Autodesk Fusion 360 part; units mm, degrees
sketch "草图1" plane through (0, 0, 0) normal (0, 0, 1) x (1, 0, 0)
  line L0 (-100, 87.5) -> (100, 87.5)
  line L1 (100, 87.5) -> (100, -87.5)
  line L2 (100, -87.5) -> (-100, -87.5)
  line L3 (-100, -87.5) -> (-100, 87.5)
  line L4 (-100, 0) -> (100, 0) construction
  line L5 (0, 75) -> (0, -50) construction
  dimension "d1" = 200
  dimension "d2" = 175
extrude "拉伸1" add sketch "草图1" against normal blind 100
sketch "草图2" plane through (0, -87.5, 0) normal (0, -1, 0) x (1, 0, 0)
  line L0 (100, 0) -> (-100, 0)
  line L1 (-100, 0) -> (-100, -100)
  line L2 (-100, -100) -> (100, -100)
  line L3 (100, -100) -> (100, 0)
  circle A0 centre (0, 0) radius 50
  dimension "d5" = 100
extrude "拉伸2" cut sketch "草图2" against normal blind 100 contours L0 A0 picked at (10.3915, -13.0305)
sketch "草图3" plane through (100, 0, 0) normal (1, 0, 0) x (0, 1, 0)
  line L0 (87.5, 0) -> (-87.5, 0)
  line L1 (-87.5, 0) -> (-87.5, -100)
  line L2 (-87.5, -100) -> (87.5, -100)
  line L3 (87.5, -100) -> (87.5, 0)
  line L4 (87.5, 0) -> (312.5, -75)
  line L5 (312.5, -75) -> (312.5, -100)
  line L6 (312.5, -100) -> (87.5, -100)
  line L7 (-150, 0) -> (245.1978, 0) construction
  dimension "d8" = 25
  dimension "d9" = 225
extrude "拉伸3" add sketch "草图3" against normal blind 100 contours L3 L4 L5 L6
sketch "草图4" plane through (-100, 0, 0) normal (-1, 0, 0) x (0, -1, 0)
  line L0 (87.5, 0) -> (-87.5, 0)
  line L1 (-87.5, 0) -> (-87.5, -100)
  line L2 (-87.5, -100) -> (87.5, -100)
  line L3 (87.5, -100) -> (87.5, 0)
  line L4 (-312.5, 75) -> (-87.5, 0)
  line L5 (-87.5, -100) -> (-312.5, -100)
  line L6 (-312.5, -100) -> (-312.5, 75)
  dimension "d12" = 175
  dimension "d13" = 225
extrude "拉伸4" add sketch "草图4" against normal blind 100 contours L1 L4 L5 L6
ref_plane "工作平面1" through (0, 0, 100) normal (0, 0, 1) x (1, 0, 0)
sketch "草图5" plane through (0, 0, 100) normal (0, 0, 1) x (1, 0, 0)
  line L0 (-50, 312.5) -> (50, 312.5)
  line L1 (50, 312.5) -> (0, 37.5)
  line L2 (0, 37.5) -> (-50, 312.5)
  line L3 (0, -125) -> (0, 391.0284) construction
  point P0 (100, -87.5)
  point P1 (-100, -87.5)
  point P2 (-100, 87.5)
  point P3 (100, 87.5)
  point P4 (-100, 312.5)
  point P5 (100, 312.5)
  dimension "d17" = 275
  dimension "d18" = 100
extrude "拉伸5" add sketch "草图5" against normal through all
sketch "草图6" plane through (100, 0, 0) normal (1, 0, 0) x (0, 1, 0)
  line L0 (87.5, 0) -> (-87.5, 0)
  line L1 (-87.5, 0) -> (-87.5, -100)
  line L2 (-87.5, -100) -> (312.5, -100)
  line L3 (312.5, -100) -> (312.5, -75)
  line L4 (312.5, -75) -> (87.5, 0)
  line L5 (37.5, 100) -> (37.5, 93.4578)
  line L6 (37.5, 93.4578) -> (37.5, 75)
  line L7 (37.5, 75) -> (312.5, 100)
  line L8 (312.5, 100) -> (37.5, 100)
  point P0 (37.5, 100)
  point P1 (312.5, 100)
  dimension "d20" = 25
extrude "拉伸6" cut sketch "草图6" against normal blind 375 contours L5 L6 L7 L8
equation "d2 = 400 mm - 225 mm"
Read the model definition and answer for the solid it produces. Units are mm, in the model's axes. A direction names the side the tool comes from. Give positions to 0.01 mm unless a question says otherwise; leave off trailing zeros. Write each loop counter-clockwise with the first axis right and the second up, starting at its lowest first coordinate (ties: lowest second). Pieces come first, ordered by that corner, then holes. Notation, with made-up numbers: (1, 38) - (48, 38) arc R18 cw to (48, 69) - close; hole circle Ø7 at (-21.5, 27). An arc over 180 degrees is marked (long way). Return JSON: item names as keys, results as strings.
Q1. A cutting plane is placed at C-C, the plane z = -46. Determine the outline of the cut face in (x, y).
Reply:
{"outline": "(-100, -87.5) - (-19.6, -87.5) - (-19.6, 12.5) - (19.6, 12.5) - (19.6, -87.5) - (100, -87.5) - (100, 225.5) - (34.18, 225.5) - (50, 312.5) - (-100, 312.5) - close"}
Q2. A cutting plane is placed at B-B, the plane x = 28.5. Determine the outline of the cut face in (y, z).
Reply:
{"outline": "(-87.5, -100) - (194.25, -100) - (194.25, -101) - (312.5, -101) - (312.5, 100) - (194.25, 89.25) - (194.25, -35.58) - (87.5, 0) - (12.5, 0) - (12.5, -41.08) - (-87.5, -41.08) - close"}
Q3. For a pull along Y with two mould halves and no side action, classify faces 1 (the face through (-1, 21, 0)), 2 (the face through (25.35, 176.92, -100.49)), 3 (the face through (65.283, 198.425, -36.975)), 4 (the face through (30.906, 207.481, 33.169)) as released by +Y, released by -Y, zero draft, split by the parting line, or undercut.
Reply:
{"face 1": "zero draft", "face 2": "released by -Y", "face 3": "undercut", "face 4": "undercut"}
Q4. For faces 5 (the face through (-1.099, -38.2, -49.988)), 6 (the face through (-24, 110, -100)), 7 (the face through (-24.65, 173.08, -100.49)), 8 (the face through (-65.283, 201.575, 38.025)), determine the directions among +Z, -Z, +X, -X, +Y, -Y from which every point of the face is accessible in a straight line to the end or side of a thin tool.
Reply:
{"face 5": "+Z, -Y", "face 6": "-Z, -Y", "face 7": "-Z, -X, -Y", "face 8": "+Z, -X, -Y"}
Q5. Consider line 1 along Z through (x, y) = (11, 33); line 2 along Y through (x, z) = (19.5, -46); line 3 along Z through (x, y) = (-3, -48). Determine where each line is inside the solid, lowest interval first. Write a range as [from, to].
Reply:
{"line 1": "[-100, 0]", "line 2": "[12.5, 312.5]", "line 3": "[-100, -49.91]"}
Q6. A cutting plane is placed at D-D, the plane z = -5. Determine the outline of the cut face in (x, y).
Reply:
{"outline": "(-100, -87.5) - (-49.75, -87.5) - (-49.75, 12.5) - (49.75, 12.5) - (49.75, -87.5) - (100, -87.5) - (100, 102.5) - (11.82, 102.5) - (50, 312.5) - (-100, 312.5) - close"}
Q7. Given P1, Ø3, axis at x = 57.5, y = 245.5, coming from the +Z side; P2, Ø5, axis at x = 75, y = 114.5, coming from the -Z side; P3, Ø8, axis at x = 17.5, y = 125.5, coming from the +Z side, each flat-ended and moving along its own axis, determine where each tip first touches the part or whether it passes through.
Reply:
{"P1": "z = -52.17", "P2": "z = -100", "P3": "z = 83.36"}
Q8. A cutting plane is placed at A-A, the plane y = 58. Determine the outline of the cut face in (x, z), and give its area (3 significant figures).
Reply:
{"outline": "(-100, -100) - (-3.73, -100) - (-3.73, -101) - (3.73, -101) - (3.73, -100) - (100, -100) - (100, 0) - (3.73, 0) - (3.73, 76.86) - (-3.73, 76.86) - (-3.73, 0) - (-100, 0) - close", "area": "20,600 mm²"}
